Solid Edge part; units mm, degrees
sketch "Sketch1" plane through (0, 0, 0) normal (0, 0, 1) x (1, 0, 0)
  line L0 (83.1, 37.5) -> (65.55, 37.5)
  line L1 (65.55, 37.5) -> (65.55, 86.5)
  line L2 (65.55, 86.5) -> (17.55, 86.5)
  line L3 (17.55, 86.5) -> (17.55, 37.5)
  line L4 (0, 37.5) -> (17.55, 37.5)
  line L5 (0, 0) -> (0, 37.5)
  line L6 (0, 0) -> (83.1, 0)
  line L7 (83.1, 0) -> (83.1, 37.5)
extrude "Protrusion1" add sketch "Sketch1" along normal blind 4
sketch "Sketch2" plane through (40.5, 43.25, 4) normal (0, 0, 1) x (1, 0, 0)
  line L0 (-29.5, -5.75) -> (-29.5, -43.25)
  line L1 (-29.5, -43.25) -> (-40.5, -43.25)
  line L2 (-40.5, -43.25) -> (-40.5, -5.75)
  line L3 (-40.5, -5.75) -> (-29.5, -5.75)
  line L4 (-20.53, -43.25) -> (-20.53, -11.85)
  line L5 (-20.53, -11.85) -> (-19.23, -11.85)
  line L6 (-19.23, -11.85) -> (-19.23, -43.25)
  line L7 (-19.23, -43.25) -> (-20.53, -43.25)
  line L8 (-16.73, -11.85) -> (-16.73, -43.25)
  line L9 (-16.73, -43.25) -> (-18.03, -43.25)
  line L10 (-18.03, -43.25) -> (-18.03, -11.85)
  line L11 (-18.03, -11.85) -> (-16.73, -11.85)
  line L12 (18.83, -11.85) -> (18.83, -43.25)
  line L13 (18.83, -43.25) -> (20.13, -43.25)
  line L14 (20.13, -43.25) -> (20.13, -11.85)
  line L15 (20.13, -11.85) -> (18.83, -11.85)
  line L16 (22.63, -43.25) -> (22.63, -11.85)
  line L17 (22.63, -11.85) -> (21.33, -11.85)
  line L18 (21.33, -11.85) -> (21.33, -43.25)
  line L19 (21.33, -43.25) -> (22.63, -43.25)
  line L20 (31.6, -5.75) -> (31.6, -43.25)
  line L21 (31.6, -43.25) -> (42.6, -43.25)
  line L22 (42.6, -43.25) -> (42.6, -5.75)
  line L23 (42.6, -5.75) -> (31.6, -5.75)
extrude "ExtrudedProtrusion_2" add sketch "Sketch2" along normal blind 2
sketch "Sketch3" plane through (41.55, 43.25, 4) normal (0, 0, 1) x (1, 0, 0)
  line L0 (-12.58, -11.85) -> (19.08, -11.85)
  line L1 (19.08, -11.85) -> (19.08, -3.85)
  line L2 (19.08, -3.85) -> (-12.58, -3.85)
  line L3 (-12.58, -11.85) -> (-12.58, -3.85)
extrude "ExtrudedProtrusion_3" add sketch "Sketch3" along normal blind 11.2
hole "Hole_1" at (60.63, 35.4, 11.2) direction (-1, 0, 0) diameter 4 depth 5.9
sketch "Sketch4" plane through (41.55, 43.25, 4) normal (0, 0, 1) x (1, 0, 0)
  line L0 (12.5, 34.25) -> (-12.5, 34.25)
  line L1 (-12.5, 34.25) -> (-12.5, 39.25)
  line L2 (-12.5, 39.25) -> (12.5, 39.25)
  line L3 (12.5, 39.25) -> (12.5, 34.25)
  line L4 (-17.5, 26.75) -> (17.5, 26.75)
  line L5 (17.5, 26.75) -> (17.5, 6.75)
  line L6 (17.5, 6.75) -> (-17.5, 6.75)
  line L7 (-17.5, 6.75) -> (-17.5, 26.75)
extrude "Cutout1" cut sketch "Sketch4" against normal through all
hole "Hole_3" at (7, 6, 0) direction (0, 0, 1) diameter 3 end through all countersink diameter 6.94 countersink angle 90
hole "Hole1" at (7, 25.5, 0) direction (0, 0, 1) diameter 3 end through all countersink diameter 6.94 countersink angle 90
hole "Hole2" at (76.1, 6, 0) direction (0, 0, 1) diameter 3 end through all countersink diameter 6.94 countersink angle 90
hole "Hole3" at (76.1, 25.5, 0) direction (0, 0, 1) diameter 3 end through all countersink diameter 6.94 countersink angle 90
sketch "Sketch5" plane through (41.55, 15.7, 4) normal (0, 0, 1) x (1, 0, 0)
  line L0 (-8.0007, -13.7) -> (7.9993, -13.7)
  line L1 (7.9993, -13.7) -> (7.9993, -15.7)
  line L2 (-8.0007, -15.7) -> (7.9993, -15.7)
  line L3 (-8.0007, -13.7) -> (-8.0007, -15.7)
extrude "ExtrudedProtrusion_4" add sketch "Sketch5" along normal blind 1
fillet "Round_1" radius 0.6 2 edges at (41.5493, 2, 5) (41.5493, 0, 5)
sketch "Sketch6" plane through (41.55, 31.4, 9.6) normal (0, -1, 0) x (1, 0, 0)
  line L0 (-4.92, 0.65) -> (-4.92, -2.35)
  line L1 (-4.92, -2.35) -> (13.08, -2.35)
  line L2 (13.08, -2.35) -> (13.08, 0.65)
  line L3 (13.08, 0.65) -> (-4.92, 0.65)
extrude "ExtrudedCutout_2" cut sketch "Sketch6" against normal blind 2.8
sketch "Sketch7" plane through (41.55, 39.4, 9.6) normal (0, 1, 0) x (-1, 0, 0)
  line L0 (-13.08, 0.65) -> (4.92, 0.65)
  line L1 (4.92, 0.65) -> (4.92, -2.35)
  line L2 (4.92, -2.35) -> (-13.08, -2.35)
  line L3 (-13.08, -2.35) -> (-13.08, 0.65)
extrude "ExtrudedCutout_5" cut sketch "Sketch7" against normal blind 3
sketch "Sketch8" plane through (39.36, 34.2, 9.93) normal (0, -1, 0) x (1, 0, 0)
  line L0 (-2.41, -0.23) -> (15.09, -0.23)
  line L1 (15.09, -0.23) -> (15.09, -2.23)
  line L2 (15.09, -2.23) -> (-2.41, -2.23)
  line L3 (-2.41, -2.23) -> (-2.41, -0.23)
extrude "Cutout2" cut sketch "Sketch8" against normal up to next
sketch "Sketch9" plane through (40.5, 43.25, 4) normal (0, 0, 1) x (1, 0, 0)
  line L0 (-11.53, -24.85) -> (-11.53, -11.85)
  line L1 (-11.53, -11.85) -> (-12.53, -11.85)
  line L2 (-12.53, -11.85) -> (-12.53, -24.85)
  line L3 (-12.53, -24.85) -> (-11.53, -24.85)
extrude "ExtrudedCutout_7" cut sketch "Sketch9" against normal blind 0.7
sketch "Sketch10" plane through (41.55, 35.4, 15.2) normal (0, 0, 1) x (1, 0, 0)
  line L0 (-13.58, 4) -> (-13.58, -4)
  line L1 (-13.58, -4) -> (-12.58, -4)
  line L2 (-12.58, -4) -> (-12.58, 4)
  line L3 (-12.58, 4) -> (-13.58, 4)
extrude "ExtrudedCutout_8" cut sketch "Sketch10" against normal blind 11.9
fillet "Round_2" radius 0.1 1 edges at (36.95, 34.2, 8.7)
fillet "Round_3" radius 0.1 7 edges at (54.45, 36.4, 8.7) (36.95, 36.4, 8.7) (45.7, 36.4, 7.7) (45.7, 36.4, 9.7) (45.65, 34.2, 7.7) (54.45, 34.2, 8.7) (45.65, 34.2, 9.7)
hole "Hole_7" at (28.97, 35.4, 11.2) direction (1, 0, 0) diameter 4 depth 6
Geometry check sheet. Reference: the model listing, model coordinates, mm. A direction names the side the tool comes from. Give positions to 0.01 mm unless a question says otherwise; leave off trailing zeros. Loops run counter-clockwise (first coordinate to the right, second up) from the corner with the lowest first, then second, coordinate; pieces in that order, holes last. Notation, with made-up numbers: M -30,40 L -19,40 A25 ccw -19,55 Z; hole C 0,-20.75 d5. An arc over 180 degrees is marked long. Answer as CSV lines item,"result".
Item 1: Depth check by flat-ended pin: P1, Ø1.5, axis at x = 22, y = 10.5, coming from the -Z side; P2, Ø3, axis at y = 35.4, z = 11.2, coming from the +X side; P3, Ø0.9, axis at y = 38, z = 8.5, coming from the -X side; P4, Ø5, axis at x = 36.5, y = 13, coming from the +Z side. Enter the tip coordinate at first touch or a pass-through.
Values:
P1,"stops at z = 0"
P2,"stops at x = 54.73"
P3,"stops at x = 28.97"
P4,"stops at z = 4"
Item 2: Release check for a two-part mould opening along Z. For faces 1 (the flat face through (46, 38, 10.25)), 2 (the conical face through (6.378, 26.999, 1.847)), 3 (the cylindrical face through (74.77, 6.69, 3.96)) record: pulls with the +Z half, pulls with the -Z half, needs draft (parallel to the pull), parting line crosses it, or undercut.
Values:
face 1,"undercut"
face 2,"pulls with the -Z half"
face 3,"needs draft"
Item 3: Cross-section at B-B on x = 7. Record the cut outline in (y, z), and give its area (3 significant figures).
Values:
outline,"M 0,0 L 2.53,0 L 4.5,1.97 L 4.5,6 L 0,6 Z; M 7.5,1.97 L 9.47,0 L 22.03,0 L 24,1.97 L 24,6 L 7.5,6 Z; M 27,1.97 L 28.97,0 L 37.5,0 L 37.5,6 L 27,6 Z"
area,"181 mm²"
Item 4: Access from +Z, -Z, +X, -X, +Y, -Y to the whole of each face (thin tool, end or side, straight path). Record for faces 4 (the flat face through (17.55, 62, 2)), 5 (the cylindrical face through (57.639, 36.166, 9.353)), 6 (the flat face through (41, 82.5, 2)), 7 (the flat face through (36.63, 38, 9)).
Values:
face 4,"+Z, -Z, -X, +Y"
face 5,"+X"
face 6,"+Z, -Z"
face 7,"+Y"
Item 5: Material ranges on line 1 (Z direction, x = 57.3, y = 35.4); line 2 (Y direction, x = 7, z = 3.15); line 3 (Y direction, x = 42, z = 4.25), recorded low to high.
Values:
line 1,"z = 0 to 9.2, 13.2 to 15.2"
line 2,"y = 0 to 4.5, 7.5 to 24, 27 to 37.5"
line 3,"y = 0 to 2, 31.4 to 39.4"
Item 6: Cross-section at A-A on y = 54. Record the cut outline in (x, z).
Values:
outline,"M 17.55,0 L 24.05,0 L 24.05,4 L 17.55,4 Z; M 59.05,0 L 65.55,0 L 65.55,4 L 59.05,4 Z"
Item 7: Cross-section at C-C on z = 1. Record the cut outline in (x, y), and give its area (3 significant figures).
Values:
outline,"M 0,0 L 83.1,0 L 83.1,37.5 L 65.55,37.5 L 65.55,86.5 L 17.55,86.5 L 17.55,37.5 L 0,37.5 Z; hole C 7,6 d4.94; hole C 7,25.5 d4.94; hole M 24.05,50 L 59.05,50 L 59.05,70 L 24.05,70 Z; hole M 29.05,77.5 L 54.05,77.5 L 54.05,82.5 L 29.05,82.5 Z; hole C 76.1,6 d4.94; hole C 76.1,25.5 d4.94"
area,"4,570 mm²"
Item 8: Cross-section at D-D on y = 15. Record the cut outline in (x, z).
Values:
outline,"M 0,0 L 83.1,0 L 83.1,6 L 72.1,6 L 72.1,4 L 63.13,4 L 63.13,6 L 61.83,6 L 61.83,4 L 60.63,4 L 60.63,6 L 59.33,6 L 59.33,4 L 23.77,4 L 23.77,6 L 22.47,6 L 22.47,4 L 21.27,4 L 21.27,6 L 19.97,6 L 19.97,4 L 11,4 L 11,6 L 0,6 Z"
